The model under review builds one solid part; all positions refer to its coordinate system, in mm. A direction names the side the tool comes from. Coordinates: 2 decimals unless noted, no trailing zeros. Write each loop counter-clockwise with the first axis right and the second up, starting at its lowest first coordinate (ties: lowest second). Pieces come first, ordered by that corner, then holes. Notation, with made-up numbers: (48.5, -23) - (66.5, -23) arc R30 cw to (66.5, 9) - close; hole circle Ø4 at (87.5, 76.25). An arc over 180 degrees is marked (long way). Put each result on its own line as item: value. Start each with the question number.
Item 1: Consider section C-C on y = 5.75. Give the boundary of the cut face in (x, z), then the cut area to 3 significant figures.
Item 2: Consider section A-A on y = 11. Give the boundary of the cut face in (x, z).
Item 3: Consider section D-D on z = 59. Give the boundary of the cut face in (x, y).
Item 4: Mouldability with a two-part tool opening along X and no side actions: class faces 3 (the face through (32.18, 13.23, 50.47)), 4 (the face through (37, 10, 91)), 5 (the face through (37.08, 4.13, 3.75)) as pulls with the +X half, pulls with the -X half, needs draft (parallel to the pull), parting line crosses it, or undercut.
Item 5: To check wall thickness, follow L1, parallel to Z at x = 40.75, y = 3.75; L2, parallel to Z at x = 37.5, y = 4.75; L3, parallel to X at y = 8, z = -6. State the ranges of each line that lie inside material, in increasing order. Write a range as [from, to].
Item 6: Consider section B-B on x = 46.25. Give the boundary of the cut face in (y, z), then the cut area to 3 significant figures.
Item 7: Machinability: for faces 1 (the face through (37, 10, 0)), 2 (the face through (31, 0, -6)), which of the approach directions +Z, -Z, +X, -X, +Y, -Y give a long, thin tool a straight path to every point of the face, cutting with its end or side? Answer none if there is none.
Item 8: For pin 1 (9.5 mm diameter, centred on x = 39.5, y = 11, fed in from -Z); pin 2 (3 mm diameter, centred on x = 32, z = 68.5, fed in from -Y); pin 3 (1 mm diameter, centred on x = 31, y = 10.5, fed in from -Z), all flat-tipped, find the tip position at first contact; note any pin that passes through.
```python
from build123d import *

# Parameters (mm, degrees)
SKETCH2_R           = 6
BOSS_EXTRUDE1_DEPTH = 91


with BuildPart() as part:
    # Sketch1 → Revolve1 (revolve)
    with BuildSketch(Plane.XY, mode=Mode.PRIVATE) as revolve1_sk:
        with BuildLine():
            ThreePointArc((37.312583507, 16), (28.368311597, 10.472135955), (29.312583507, 0))
            Line((29.312583507, 0), (23.564856422, 0))
            ThreePointArc((23.564856422, 0), (24.762683109, 14.215838363), (37.312583507, 21))
            Line((37.312583507, 21), (37.312583507, 16))
        make_face()
    revolve(revolve1_sk.sketch.rotate(Axis((37.312583507, 21, 0), (0, -1, 0)), 180), axis=Axis((37.312583507, 21, 0), (0, -1, 0)))

    # Sketch2 → Boss-Extrude1 (add)
    with BuildSketch(Plane.XY):
        with Locations(Location((37.312583507, 10.123565848, 0), (0, 0, 211.358745585))):
            Circle(SKETCH2_R)
    extrude(amount=BOSS_EXTRUDE1_DEPTH)


solid = part.part
```
Report:
1. outline: (33.21, 14.42) arc R15 ccw (long way) to (41.42, 14.42) - (41.42, 91) - (33.21, 91) - close; hole (33.21, 0) - (33.21, 9.11) arc R10 ccw (long way) to (41.42, 9.11) - (41.42, 0) - close
1. area: 1,100 mm²
2. outline: (31.38, 12.84) arc R14.14 ccw (long way) to (43.25, 12.84) - (43.25, 91) - (31.38, 91) - close; hole (31.38, 0) - (31.38, 6.31) arc R8.66 ccw (long way) to (43.25, 6.31) - (43.25, 0) - close
3. outline: circle Ø12 at (37.31, 10.12)
4. face 3: parting line crosses it
4. face 4: needs draft
4. face 5: undercut
5. L1: [-14.43, -9.12], [9.12, 14.43]
5. L2: [-14.95, -9.92], [0, 91]
5. L3: [23.71, 29.57], [45.06, 50.91]
6. outline: (0, -10.45) arc R12.05 ccw (long way) to (0, 10.45) - close; hole circle Ø8.97 at (6, 0)
6. area: 303 mm²
7. face 1: -Y
7. face 2: +Z, -Z, +X, -X, -Y
8. pin 1: z = -14.98
8. pin 2: y = 5.49
8. pin 3: z = -13.13
